from build123d import *

# Parameters (mm, degrees)
ESQUISSE1_R                  = 60
BOSS_EXTRU_1_DEPTH           = 10
ESQUISSE2_R                  = 7.5
BOSS_EXTRU_2_DEPTH           = 15
R_P_TITION_CIRCULAIRE1_COUNT = 6


with BuildPart() as part:
    # Esquisse1 → Boss.-Extru.1 (new body)
    with BuildSketch(Plane(origin=(0, 0, 0), x_dir=(1, 0, 0), z_dir=(0, 1, 0))):
        with Locations(Location((0, 0, 0), (0, 0, 270))):
            Circle(ESQUISSE1_R)
    extrude(amount=BOSS_EXTRU_1_DEPTH)

    # Esquisse2 → Boss.-Extru.2 (add)
    with BuildSketch(Plane(origin=(0, 10, 0), x_dir=(1, 0, 0), z_dir=(0, 1, 0))):
        with Locations(Location((0, 45, 0), (0, 0, 270))):
            Circle(ESQUISSE2_R)
    boss_extru_2 = extrude(amount=BOSS_EXTRU_2_DEPTH)

    # Répétition circulaire1: Boss.-Extru.2 ×6 about axis
    r_p_tition_circulaire1_axis = Axis((0, 0, 0), (0, 1, 0))
    for i in range(1, R_P_TITION_CIRCULAIRE1_COUNT):
        add(boss_extru_2.rotate(r_p_tition_circulaire1_axis, i * 360 / R_P_TITION_CIRCULAIRE1_COUNT))


solid = part.part
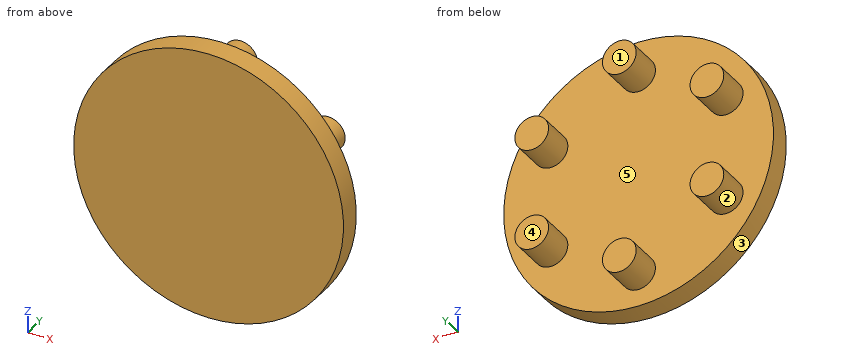
Build history of the part. All positions in model axes, mm. Face numbers are marked on the shaded views. A direction names the side the tool comes from. Give positions to 0.01 mm unless a question says otherwise; leave off trailing zeros. Order: outer loops, then holes, each group sorted by start corner. A loop starts at its lowest first (then second) coordinate and runs counter-clockwise, first axis right, second up. Notation, with made-up numbers: M 24,12.25 L 31,12.25 A11 ccw 31,23.25 Z; hole C 71,55.5 d2. An arc over 180 degrees is marked long. Put each result on its own line as item: value.
Item 1: Pull direction Z, two halves, no side cores. Call the marked faces 3, 4 and 5: +Z half, -Z half, draft (parallel to the pull), parting line (faces both ways), or undercut.
Results are:
face 3: parting line
face 4: draft
face 5: undercut
Item 2: Cut at C-C on y = 5. Write the cut outline in (x, z), then the cut area to 3 significant figures.
Results are:
outline: C 0,0 d120
area: 11,300 mm2
Item 3: Cut at A-A on x = 0. Write the cut outline in (y, z), then the cut area to 3 significant figures.
Results are:
outline: M 0,-60 L 10,-60 L 10,-52.5 L 25,-52.5 L 25,-37.5 L 10,-37.5 L 10,37.5 L 25,37.5 L 25,52.5 L 10,52.5 L 10,60 L 0,60 Z
area: 1,650 mm2
Item 4: Cut at B-B on z = -45. Write the cut outline in (x, y).
Results are:
outline: M -39.69,0 L 39.69,0 L 39.69,10 L 7.5,10 L 7.5,25 L -7.5,25 L -7.5,10 L -39.69,10 Z
Item 5: Which spindle directions (+Z, -Z, +X, -X, +Y, -Y) get a long thin tool onto all of the face, cutting with end or side? Do the marked faces 1 and 2. Say none if no direction does.
Results are:
face 1: +Z, -Z, +X, -X, +Y
face 2: +Y
Item 6: Cut at D-D on z = 27.5. Write the cut outline in (x, y), then the cut area to 3 significant figures.
Results are:
outline: M -53.33,0 L 53.33,0 L 53.33,10 L 44.56,10 L 44.56,25 L 33.38,25 L 33.38,10 L -33.38,10 L -33.38,25 L -44.56,25 L -44.56,10 L -53.33,10 Z
area: 1,400 mm2
Item 7: Drop flat-ended pins along their axis: pin 1 Ø12 at (x, y) = (14, 5) entering from -Z; pin 2 Ø6 at (y, z) = (5.5, -23.5) entering from -X; pin 3 Ø1 at (y, z) = (6, 47.5) entering from +X. Give the stop position or say it passes through.
Results are:
pin 1: z = -59.46
pin 2: x = -56.39
pin 3: x = 37.3
Item 8: Wall check: probe 1 along Y at (x, z) = (31, -33.5); probe 2 along Z at (x, y) = (0.5, 9.75); probe 3 along X at (y, z) = (23.25, 27.5). Give the ranges that are in metal, low to high.
Results are:
probe 1: 0 to 10
probe 2: -60 to 60
probe 3: -44.56 to -33.38, 33.38 to 44.56
